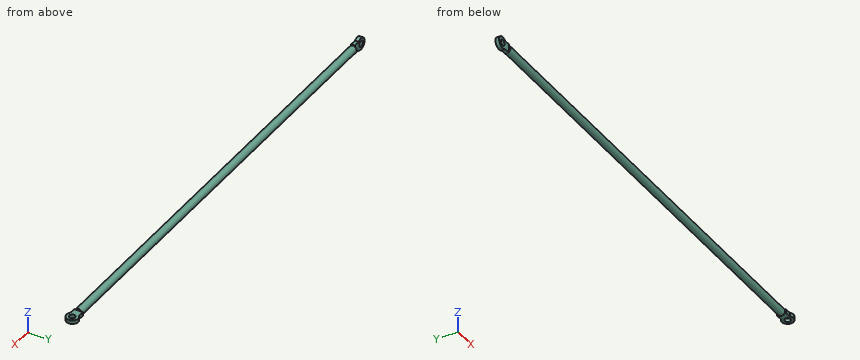
```python
from build123d import *

# Parameters (mm, degrees)
F0_R     = 5
F1_DEPTH = 620
F2_R     = 4
F3_DEPTH = 2.5
F4_R     = 4
F5_DEPTH = 2.5


with BuildPart() as f1:
    # F0 (on Right) → F1 (new body)
    with BuildSketch(Plane.YZ):
        Circle(F0_R)
    extrude(amount=F1_DEPTH)

    # F2 (on Front) → F3 (join, symmetric)
    with BuildSketch(Plane.XZ):
        with BuildLine():
            Line((0, -6), (0, 6))
            Line((0, 6), (-8.708497, 6))
            ThreePointArc((-8.708497, 6), (-22, 0), (-8.708497, -6))
            Line((-8.708497, -6), (0, -6))
        make_face()
        with Locations((-14, 0)):
            Circle(F2_R, mode=Mode.SUBTRACT)
    extrude(amount=F3_DEPTH, both=True)

    # F4 (on Top) → F5 (join, symmetric)
    with BuildSketch(Plane.XY):
        with BuildLine():
            Line((628.708497, 6), (620, 6))
            Line((620, 6), (620, -6))
            Line((620, -6), (628.708497, -6))
            ThreePointArc((628.708497, -6), (642, 0), (628.708497, 6))
        make_face()
        with Locations((634, 0)):
            Circle(F4_R, mode=Mode.SUBTRACT)
    extrude(amount=F5_DEPTH, both=True)


solid = f1.part
```
Design review of the part built by this model. Coordinates are the model's own, in mm. Give positions to 0.01 mm unless a question says otherwise; leave off trailing zeros. Order: outer loops, then holes, each group sorted by start corner. A loop starts at its lowest first (then second) coordinate and runs counter-clockwise, first axis right, second up. Notation, with made-up numbers: M 39,-19 L 98,-19 A28 ccw 98,3 Z; hole C 84,-18 d11. An arc over 180 degrees is marked long. One line per question, with ' | ' between items. Start each with the question number.
Q1. We need section B-B (x = 81). Write out the cut boundary in (y, z).
Q2. For pin 1 Ø5.5 at (x, y) = (-4, -0.5) entering from -Z; pin 2 Ø5.5 at (x, z) = (625.5, 1) entering from -Y; pin 3 Ø5 at (x, z) = (-11.5, 1.5) entering from +Y; pin 4 Ø3 at (y, z) = (0.5, -3.5) entering from +X, all flat-tipped, find the tip position at first contact; note any pin that passes through.
Q3. For L1, parallel to Z at x = -14, y = 0.1; L2, parallel to Y at x = 67, z = -0.25; L3, parallel to Z at x = 135, y = 3, list the stretches that pass through material, from the lowest coordinate up. Write a range as [from, to].
Q4. We need section A-A (y = 0). Write out the cut boundary in (x, z), plus the area to 3 significant figures.
Returned:
1) outline: C 0,0 d10
2) pin 1: z = -6 | pin 2: y = -6 | pin 3: y = 2.5 | pin 4: x = 642
3) L1: [-8, -4], [4, 8] | L2: [-4.99, 4.99] | L3: [-4, 4]
4) outline: M -8.71,-6 L 0,-6 L 0,-5 L 620,-5 L 620,-2.5 L 630,-2.5 L 630,2.5 L 620,2.5 L 620,5 L 0,5 L 0,6 L -8.71,6 A8 ccw long Z; M 638,-2.5 L 642,-2.5 L 642,2.5 L 638,2.5 Z; hole C -14,0 d8 | area: 6,500 mm2
